from build123d import *

# Parameters (mm, degrees)
F1_DEPTH = 55
F2_R     = 29
F2_R_2   = 11.5
F3_DEPTH = 6
F5_R     = 2.5
F7_DEPTH = 100
F8_COUNT = 6


with BuildPart() as f1:
    # F0 (on Top) → F1 (new body)
    with BuildSketch(Plane.XY):
        with BuildLine():
            Line((-2, -22.2686017747), (-2, -20.3608079407))
            ThreePointArc((-2, -20.3608079407), (-2.4554799552, -19.0901947694), (-3.6144578313, -18.3983204284))
            ThreePointArc((-3.6144578313, -18.3983204284), (-9.375, -16.237976321), (-14.1261839623, -12.329372517))
            ThreePointArc((-14.1261839623, -12.329372517), (-15.3048536558, -11.6716054044), (-16.6329769183, -11.9124547779))
            Line((-16.6329769183, -11.9124547779), (-18.2851748436, -12.8663516949))
            ThreePointArc((-18.2851748436, -12.8663516949), (-19.2553429626, -14.2542548846), (-18.8131461005, -15.888869022))
            ThreePointArc((-18.8131461005, -15.888869022), (-12.3125, -21.3258755682), (-4.3535911602, -24.2370969592))
            ThreePointArc((-4.3535911602, -24.2370969592), (-2.7168753608, -23.8027436065), (-2, -22.2686017747))
        make_face()
    extrude(amount=F1_DEPTH)



with BuildPart() as f1b:
    # F0 (on Top) → F1, piece 2 (new body)
    with BuildSketch(Plane.XY):
        with BuildLine():
            ThreePointArc((14.1261839623, -12.329372517), (9.375, -16.237976321), (3.6144578313, -18.3983204284))
            ThreePointArc((3.6144578313, -18.3983204284), (2.4554799552, -19.0901947694), (2, -20.3608079407))
            Line((2, -20.3608079407), (2, -22.2686017747))
            ThreePointArc((2, -22.2686017747), (2.7168753608, -23.8027436065), (4.3535911602, -24.2370969592))
            ThreePointArc((4.3535911602, -24.2370969592), (12.3125, -21.3258755682), (18.8131461005, -15.888869022))
            ThreePointArc((18.8131461005, -15.888869022), (19.2553429626, -14.2542548846), (18.2851748436, -12.8663516949))
            Line((18.2851748436, -12.8663516949), (16.6329769183, -11.9124547779))
            ThreePointArc((16.6329769183, -11.9124547779), (15.3048536558, -11.6716054044), (14.1261839623, -12.329372517))
        make_face()
    extrude(amount=F1_DEPTH)


with BuildPart() as f1c:
    # F0 (on Top) → F1, piece 3 (new body)
    with BuildSketch(Plane.XY):
        with BuildLine():
            ThreePointArc((17.7406417936, -6.0689479114), (17.7603336111, -7.418589365), (18.6329769183, -8.4483531628))
            Line((18.6329769183, -8.4483531628), (20.2851748436, -9.4022500798))
            ThreePointArc((20.2851748436, -9.4022500798), (21.9722183234, -9.5484887219), (23.1667372608, -8.3482279372))
            ThreePointArc((23.1667372608, -8.3482279372), (24.625, 0), (23.1667372608, 8.3482279372))
            ThreePointArc((23.1667372608, 8.3482279372), (21.9722183234, 9.5484887219), (20.2851748436, 9.4022500798))
            Line((20.2851748436, 9.4022500798), (18.6329769183, 8.4483531628))
            ThreePointArc((18.6329769183, 8.4483531628), (17.7603336111, 7.418589365), (17.7406417936, 6.0689479114))
            ThreePointArc((17.7406417936, 6.0689479114), (18.75, 0), (17.7406417936, -6.0689479114))
        make_face()
    extrude(amount=F1_DEPTH)


with BuildPart() as f1d:
    # F0 (on Top) → F1, piece 4 (new body)
    with BuildSketch(Plane.XY):
        with BuildLine():
            ThreePointArc((-17.7406417936, 6.0689479114), (-17.7603336111, 7.418589365), (-18.6329769183, 8.4483531628))
            Line((-18.6329769183, 8.4483531628), (-20.2851748436, 9.4022500798))
            ThreePointArc((-20.2851748436, 9.4022500798), (-21.9722183234, 9.5484887219), (-23.1667372608, 8.3482279372))
            ThreePointArc((-23.1667372608, 8.3482279372), (-24.625, 0), (-23.1667372608, -8.3482279372))
            ThreePointArc((-23.1667372608, -8.3482279372), (-21.9722183234, -9.5484887219), (-20.2851748436, -9.4022500798))
            Line((-20.2851748436, -9.4022500798), (-18.6329769183, -8.4483531628))
            ThreePointArc((-18.6329769183, -8.4483531628), (-17.7603336111, -7.418589365), (-17.7406417936, -6.0689479114))
            ThreePointArc((-17.7406417936, -6.0689479114), (-18.75, 0), (-17.7406417936, 6.0689479114))
        make_face()
    extrude(amount=F1_DEPTH)


with BuildPart() as f1e:
    # F0 (on Top) → F1, piece 5 (new body)
    with BuildSketch(Plane.XY):
        with BuildLine():
            ThreePointArc((-3.6144578313, 18.3983204284), (-2.4554799552, 19.0901947694), (-2, 20.3608079407))
            Line((-2, 20.3608079407), (-2, 22.2686017747))
            ThreePointArc((-2, 22.2686017747), (-2.7168753608, 23.8027436065), (-4.3535911602, 24.2370969592))
            ThreePointArc((-4.3535911602, 24.2370969592), (-12.3125, 21.3258755682), (-18.8131461005, 15.888869022))
            ThreePointArc((-18.8131461005, 15.888869022), (-19.2553429626, 14.2542548846), (-18.2851748436, 12.8663516949))
            Line((-18.2851748436, 12.8663516949), (-16.6329769183, 11.9124547779))
            ThreePointArc((-16.6329769183, 11.9124547779), (-15.3048536558, 11.6716054044), (-14.1261839623, 12.329372517))
            ThreePointArc((-14.1261839623, 12.329372517), (-9.375, 16.237976321), (-3.6144578313, 18.3983204284))
        make_face()
    extrude(amount=F1_DEPTH)


with BuildPart() as f1f:
    # F0 (on Top) → F1, piece 6 (new body)
    with BuildSketch(Plane.XY):
        with BuildLine():
            ThreePointArc((14.1261839623, 12.329372517), (15.3048536558, 11.6716054044), (16.6329769183, 11.9124547779))
            Line((16.6329769183, 11.9124547779), (18.2851748436, 12.8663516949))
            ThreePointArc((18.2851748436, 12.8663516949), (19.2553429626, 14.2542548846), (18.8131461005, 15.888869022))
            ThreePointArc((18.8131461005, 15.888869022), (12.3125, 21.3258755682), (4.3535911602, 24.2370969592))
            ThreePointArc((4.3535911602, 24.2370969592), (2.7168753608, 23.8027436065), (2, 22.2686017747))
            Line((2, 22.2686017747), (2, 20.3608079407))
            ThreePointArc((2, 20.3608079407), (2.4554799552, 19.0901947694), (3.6144578313, 18.3983204284))
            ThreePointArc((3.6144578313, 18.3983204284), (9.375, 16.237976321), (14.1261839623, 12.329372517))
        make_face()
    extrude(amount=F1_DEPTH)


with BuildPart() as f1_1:
    add(f1.part)

    add(f1b.part)  # F3 merges F1b

    add(f1c.part)  # F3 merges F1c

    add(f1d.part)  # F3 merges F1d

    add(f1e.part)  # F3 merges F1e

    add(f1f.part)  # F3 merges F1f
    # F2 (on Top) → F3 (join)
    with BuildSketch(Plane.XY):
        Circle(F2_R)
        Circle(F2_R_2, mode=Mode.SUBTRACT)
    extrude(amount=-F3_DEPTH)


with BuildPart() as f7:
    # F5 (on offset) → F7 (new body)
    with BuildSketch(Plane.XY.offset(80)):
        with Locations((24.25, 0)):
            Circle(F5_R)
    extrude(amount=-F7_DEPTH)


with BuildPart() as f8_1:
    # F8: instance of F7
    add(f7.part.rotate(Axis((0, 0, 60.7173442841), (0, 0, 1)), 1 * 360 / F8_COUNT))


with BuildPart() as f8_2:
    # F8: instance of F7
    add(f7.part.rotate(Axis((0, 0, 60.7173442841), (0, 0, 1)), 2 * 360 / F8_COUNT))


with BuildPart() as f8_3:
    # F8: instance of F7
    add(f7.part.rotate(Axis((0, 0, 60.7173442841), (0, 0, 1)), 3 * 360 / F8_COUNT))


with BuildPart() as f8_4:
    # F8: instance of F7
    add(f7.part.rotate(Axis((0, 0, 60.7173442841), (0, 0, 1)), 4 * 360 / F8_COUNT))


with BuildPart() as f8_5:
    # F8: instance of F7
    add(f7.part.rotate(Axis((0, 0, 60.7173442841), (0, 0, 1)), 5 * 360 / F8_COUNT))


with BuildPart() as f1_2:
    add(f1_1.part)

    # F9: cut F7, F8_2, F8_3, F8_4, F8_5, F8_1
    add(f7.part, mode=Mode.SUBTRACT)
    add(f8_2.part, mode=Mode.SUBTRACT)
    add(f8_3.part, mode=Mode.SUBTRACT)
    add(f8_4.part, mode=Mode.SUBTRACT)
    add(f8_5.part, mode=Mode.SUBTRACT)
    add(f8_1.part, mode=Mode.SUBTRACT)


solid = f1_2.part
For this review, take the finished solid that the model builds, in its own axes (mm). A direction names the side the tool comes from. Give positions to 0.01 mm unless a question says otherwise; leave off trailing zeros. Loops run counter-clockwise (first coordinate to the right, second up) from the corner with the lowest first, then second, coordinate; pieces in that order, holes last. Notation, with made-up numbers: (-10.75, -1) - (36.25, -1) arc R14 cw to (36.25, 15) - close; hole circle Ø3 at (-12.75, 17.5). An arc over 180 degrees is marked (long way). Write each question's results on one line, items separated by ' | '.
(1) For faces 5 (the cylindrical face through (-24.003, 5.5, 27.115)), 6 (the flat face through (19.47, 8.93, 27.12)), 7 (the cylindrical face through (16.703, -18.095, 27.115)), 8 (the cylindrical face through (24.02, 5.42, 27.12)), 9 (the flat face through (-17.471, 12.396, 27.115)), list the 3-axis set-ups (+Z, -Z, +X, -X, +Y, -Y) from which the entire face can be reached by the end or side of a thin tool; tool diameter is ignored.
Conclusion:
face 5: +Z, -X, +Y | face 6: +Z | face 7: +Z, +X, -Y | face 8: +Z, +X, +Y | face 9: +Z, -X
(2) Take a section at B-B (y = 0). Give the boundary of the cut face in (x, z).
Conclusion:
outline: (-29, -6) - (-26.75, -6) - (-26.75, 0) - (-29, 0) - close; (-21.75, -6) - (-11.5, -6) - (-11.5, 0) - (-18.75, 0) - (-18.75, 55) - (-21.75, 55) - close; (11.5, -6) - (21.75, -6) - (21.75, 55) - (18.75, 55) - (18.75, 0) - (11.5, 0) - close; (26.75, -6) - (29, -6) - (29, 0) - (26.75, 0) - close
(3) Take a section at A-A (x = 0). Give the boundary of the cut face in (y, z), then the cut area to 3 significant figures.
Conclusion:
outline: (-29, -6) - (-11.5, -6) - (-11.5, 0) - (-29, 0) - close; (11.5, -6) - (29, -6) - (29, 0) - (11.5, 0) - close | area: 210 mm^2
(4) Take a section at C-C (z = 4.5). State how many separate pieces and enclosed holes the cut face has, then the cut area to 3 significant figures.
Conclusion:
separate pieces: 6 | enclosed holes: 0 | area: 569 mm^2
(5) Take a section at D-D (y = -17.5). Give the boundary of the cut face in (x, z).
Conclusion:
outline: (-23.12, -6) - (23.12, -6) - (23.12, 0) - (17.32, 0) - (17.32, 55) - (6.73, 55) - (6.73, 0) - (-6.73, 0) - (-6.73, 55) - (-17.32, 55) - (-17.32, 0) - (-23.12, 0) - close
(6) Draft analysis for pull direction X (two halves, no side actions). For faces 1 (the flat face through (2, 21, 27)), 2 (the flat face through (17.448, 12.383, 27.115)), 3 (the flat face through (-2, -21, 27)), 4 (the flat face through (21, 0, 55)), state which applies: +X half, -X half, draft (parallel to the pull), parting line (faces both ways), or undercut.
Conclusion:
face 1: undercut | face 2: +X half | face 3: undercut | face 4: draft
(7) For pin 1 Ø1.5 at (y, z) = (-21.5, 19.5) entering from +X; pin 2 Ø1.5 at (y, z) = (21, 29.5) entering from -X; pin 3 Ø10 at (x, z) = (9, 14) entering from -Y; pin 4 Ø18.5 at (x, y) = (0, 0) entering from -Z, all flat-tipped, find the tip position at first contact; note any pin that passes through.
Conclusion:
pin 1: x = 9.96 | pin 2: x = -9.74 | pin 3: y = -24.27 | pin 4: through
(8) For line 1 along X through (y, z) = (-21.5, 17.5); line 2 along Y through (x, z) = (-15.5, 30); line 3 along X through (y, z) = (-19, 30), list the stretches that pass through material, from the lowest coordinate up.
Conclusion:
line 1: -9.68 to -2, 2 to 9.68 | line 2: -19.13 to -11.65, 11.65 to 19.13 | line 3: -15.66 to -13.62, -10.63 to -2.53, 2.53 to 10.63, 13.62 to 15.66
